```python
from build123d import *

# Parameters (mm, degrees)
SKETCH1_W           = 140
SKETCH1_H           = 22
BOSS_EXTRUDE1_DEPTH = 16
SKETCH2_R           = 3
HOLES_DEPTH         = 15.8
SKETCH3_R           = 3
CUT_EXTRUDE2_DEPTH  = 76.099933422
FILLET2_R           = 2
FILLET4_R           = 2


with BuildPart() as part:
    # Sketch1 → Boss-Extrude1 (new body)
    with BuildSketch(Plane.XY):
        Rectangle(SKETCH1_W, SKETCH1_H)
    extrude(amount=BOSS_EXTRUDE1_DEPTH)

    # Sketch2 → holes (cut)
    with BuildSketch(Plane.XY.offset(16)):
        with Locations((35, 0)):
            Circle(SKETCH2_R)
        with Locations((50, 0)):
            Circle(SKETCH2_R)
        with Locations((-35, 0)):
            Circle(SKETCH2_R)
        with Locations((-50, 0)):
            Circle(SKETCH2_R)
    extrude(amount=-HOLES_DEPTH, mode=Mode.SUBTRACT)

    # Sketch3 → Cut-Extrude2 (cut, through all)
    with BuildSketch(Plane(origin=(0, 11, 0), x_dir=(1, 0, 0), z_dir=(0, 1, 0))):
        with Locations(Location((0, -8, 0), (0, 0, 270))):
            Circle(SKETCH3_R)
        with Locations(Location((60, -8, 0), (0, 0, 270))):
            Circle(SKETCH3_R)
        with Locations(Location((-60, -8, 0), (0, 0, 90))):
            Circle(SKETCH3_R)
    extrude(amount=-CUT_EXTRUDE2_DEPTH, mode=Mode.SUBTRACT)

    # Fillet2
    fillet2_edges = [part.edges().sort_by_distance(p)[0] for p in [
        (-70, -11, 8),
        (-70, 11, 8),
    ]]
    fillet(fillet2_edges, radius=FILLET2_R)

    # Fillet4
    fillet4_edges = [part.edges().sort_by_distance(p)[0] for p in [
        (70, -11, 8),
        (70, 11, 8),
    ]]
    fillet(fillet4_edges, radius=FILLET4_R)


solid = part.part
```
Geometry check sheet. Reference: the model listing, model coordinates, mm. A direction names the side the tool comes from. Round coordinates to 2 decimals unless told otherwise and drop trailing zeros. Loops run counter-clockwise (first coordinate to the right, second up) from the corner with the lowest first, then second, coordinate; pieces in that order, holes last. Notation, with made-up numbers: (-10, 85) - (28, 85) arc R15 cw to (28, 92) - close; hole circle Ø10 at (88, -8.75). An arc over 180 degrees is marked (long way). Write item = value, one per line. Start each with the question number.
1. Section check C-C on z = 1.5. Enter the section's corners in (x, y), then the cut area to 3 significant figures.
2. Section check D-D on y = 0. Enter the section's corners in (x, z), then the cut area to 3 significant figures.
3. Depth check by flat-ended pin: pin 1 (3 mm diameter, centred on x = -49.5, y = 0, fed in from +Z). Enter the tip coordinate at first touch or a pass-through.
4. Thickness scan on line 1 (X direction, y = -5.5, z = 8); line 2 (Y direction, x = 50, z = 9.75); line 3 (X direction, y = -2.75, z = 3.75). Record the ranges inside material, lowest first.
5. Section check B-B on z = 8. Enter the section's corners in (x, y).
6. Set-up check for faces 5 (the face through (70, 0, 8)), 6 (the face through (-50, 0, 0.2)): record each of +Z, -Z, +X, -X, +Y, -Y from which the full face is reachable in a straight line by a thin tool's end or side.
7. Section check A-A on x = 0. Enter the section's corners in (y, z).
8. Mould release check, pull along Y, two halves, no side actions. Record for faces 1 (the face through (-35, 0, 0.2)), 2 (the face through (-1.15, 0.15, 10.77)), 3 (the face through (-1, 11, 11)), 4 (the face through (-38, 0, 8)): released by +Y, released by -Y, zero draft, split by the parting line, or undercut.
Working result:
q1.outline = (-70, -9) arc R2 ccw to (-68, -11) - (68, -11) arc R2 ccw to (70, -9) - (70, 9) arc R2 ccw to (68, 11) - (-68, 11) arc R2 ccw to (-70, 9) - close; hole circle Ø6 at (-50, 0); hole circle Ø6 at (-35, 0); hole circle Ø6 at (35, 0); hole circle Ø6 at (50, 0)
q1.area = 2,960 mm^2
q2.outline = (-70, 0) - (70, 0) - (70, 16) - (53, 16) - (53, 0.2) - (47, 0.2) - (47, 16) - (38, 16) - (38, 0.2) - (32, 0.2) - (32, 16) - (-32, 16) - (-32, 0.2) - (-38, 0.2) - (-38, 16) - (-47, 16) - (-47, 0.2) - (-53, 0.2) - (-53, 16) - (-70, 16) - close; hole circle Ø6 at (-60, 8); hole circle Ø6 at (0, 8); hole circle Ø6 at (60, 8)
q2.area = 1,780 mm^2
q3.pin_1 = 0.2
q4.line_1 = -70 to -63, -57 to -3, 3 to 57, 63 to 70
q4.line_2 = -11 to -3, 3 to 11
q4.line_3 = -70 to -51.2, -48.8 to -36.2, -33.8 to 33.8, 36.2 to 48.8, 51.2 to 70
q5.outline = (-70, -9) arc R2 ccw to (-68, -11) - (-63, -11) - (-63, 11) - (-68, 11) arc R2 ccw to (-70, 9) - close; (-57, -11) - (-3, -11) - (-3, 11) - (-57, 11) - close; (3, -11) - (57, -11) - (57, 11) - (3, 11) - close; (63, -11) - (68, -11) arc R2 ccw to (70, -9) - (70, 9) arc R2 ccw to (68, 11) - (63, 11) - close; hole circle Ø6 at (-50, 0); hole circle Ø6 at (-35, 0); hole circle Ø6 at (35, 0); hole circle Ø6 at (50, 0)
q6.face_5 = +Z, -Z, +X, +Y, -Y
q6.face_6 = +Z
q7.outline = (-11, 0) - (11, 0) - (11, 5) - (-11, 5) - close; (-11, 11) - (11, 11) - (11, 16) - (-11, 16) - close
q8.face_1 = undercut
q8.face_2 = zero draft
q8.face_3 = released by +Y
q8.face_4 = undercut
